Geometry check sheet. Reference: drawing and pictorial views, mm from the part's lowest x, y, z. A direction names the side the tool comes from. Coordinates: 2 decimals unless noted, no trailing zeros. Loops run counter-clockwise (first coordinate to the right, second up) from the corner with the lowest first, then second, coordinate; pieces in that order, holes last. Notation, with made-up numbers: (21, 20.5) -> (54, 20.5) arc R17 ccw to (54, 50.5) -> close; hole circle Ø9 at (57, 7.25). An arc over 180 degrees is marked (long way). Use CSV: the item, a comma, the result in double quotes.
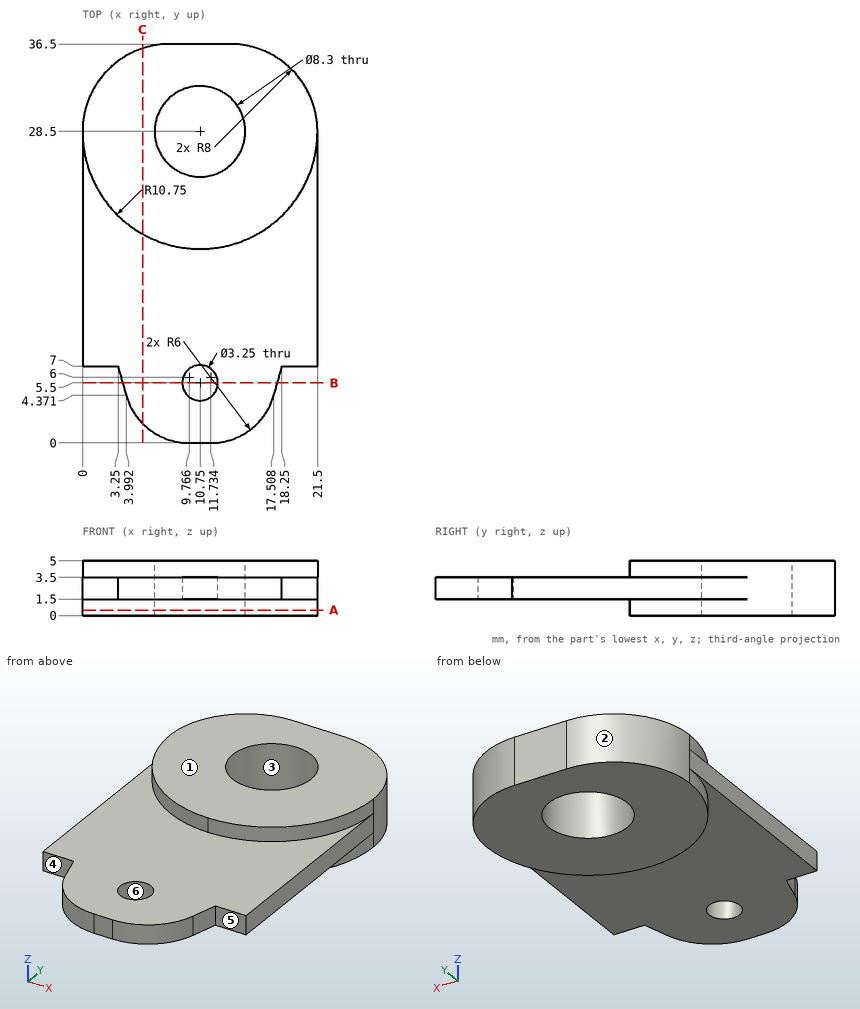
1) Cross-section at C-C on x = 5.5. Record the boundary of the cut face in (y, z).
Answer below:
outline,"(1.78, 1.5) -> (19.12, 1.5) -> (19.12, 0) -> (36.1, 0) -> (36.1, 5) -> (19.12, 5) -> (19.12, 3.5) -> (1.78, 3.5) -> close"
2) Draft check along Y on the marked faces 1, 2, 3 and 4. Enter one of: released by +Y, released by -Y, zero draft, split by the parting line, or undercut.
Answer below:
face 1,"zero draft"
face 2,"released by +Y"
face 3,"undercut"
face 4,"released by -Y"
3) Thickness scan on line 1 along Z through (x, y) = (3.25, 17); line 2 along Y through (x, z) = (7.75, 0.65) (1 decimal); line 3 along Y through (x, z) = (14.5, 4.55) (1 decimal). Record the ranges inside material, lowest first. Write a range as from..to.
Answer below:
line 1,"z = 1.5..3.5"
line 2,"y = 18.2..25.6, 31.4..36.5"
line 3,"y = 18.4..26.7, 30.3..36.4"
4) Cross-section at A-A on z = 0.5. Record the boundary of the cut face in (x, y).
Answer below:
outline,"(0, 28.5) arc R10.75 ccw to (21.5, 28.5) arc R8 ccw to (13.5, 36.5) -> (8, 36.5) arc R8 ccw to start; hole circle Ø8.3 at (10.75, 28.5)"
5) Go/stop test with flat-tipped pins: pin 1 Ø1 at (x, z) = (6, 3) entering from -Y; pin 2 Ø0.6 at (x, z) = (19.5, 3) entering from -Y; pin 3 Ø3 at (x, z) = (3, 2) entering from +Y. Record where each tip stops, or that it passes through.
Answer below:
pin 1,"stops at y = 0.97"
pin 2,"stops at y = 7"
pin 3,"stops at y = 35.69"
6) Access from +Z, -Z, +X, -X, +Y, -Y to the whole of each face (thin tool, end or side, straight path). Record for the marked faces 5 and 6.
Answer below:
face 5,"+Z, -Z, +X, -Y"
face 6,"+Z, -Z"
7) Cross-section at B-B on y = 5.5. Record the boundary of the cut face in (x, z) (1 decimal), and give its area (3 significant figures).
Answer below:
outline,"(3.7, 1.5) -> (9.1, 1.5) -> (9.1, 3.5) -> (3.7, 3.5) -> close; (12.4, 1.5) -> (17.8, 1.5) -> (17.8, 3.5) -> (12.4, 3.5) -> close"
area,"21.8 mm²"
